Here's how the part is built. I have some questions about the finished solid (model axes, mm). Face numbers are marked on the shaded views. A direction names the side the tool comes from. Round coordinates to 2 decimals unless told otherwise and drop trailing zeros. Loops run counter-clockwise (first coordinate to the right, second up) from the corner with the lowest first, then second, coordinate; pieces in that order, holes last. Notation, with made-up numbers: M -40,-18 L -8,-18 A19 cw -8,-4 Z; hole C -20,77 d3. An arc over 180 degrees is marked long. One line per question, with ' | ' between items. Start each with the question number.
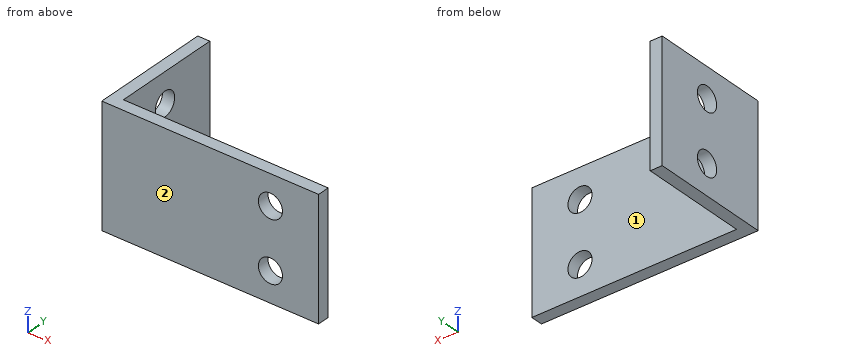
```python
from build123d import *

# Parameters (mm, degrees)
AUFSATZ_LINEAR_AUSTRAGEN1_DEPTH      = 15
AUFSATZ_LINEAR_AUSTRAGEN1_DEPTH_BACK = 15
SKIZZE5_R                            = 3
SCHNITT_LINEAR_AUSTRAGEN1_DEPTH      = 24
SKIZZE7_R                            = 3
SCHNITT_LINEAR_AUSTRAGEN2_DEPTH      = 14


with BuildPart() as part:
    # Skizze2 → Aufsatz-Linear austragen1 (new body, two sides)
    with BuildSketch(Plane.XY) as aufsatz_linear_austragen1_sk:
        Polygon((14, 51), (11, 51), (11, 21), (65, 21), (65, 24), (14, 24), align=None)
    extrude(amount=AUFSATZ_LINEAR_AUSTRAGEN1_DEPTH)
    extrude(aufsatz_linear_austragen1_sk.sketch, amount=-AUFSATZ_LINEAR_AUSTRAGEN1_DEPTH_BACK)

    # Skizze5 → Schnitt-Linear austragen1 (cut)
    with BuildSketch(Plane(origin=(0, 0, 0), x_dir=(1, 0, 0), z_dir=(0, 1, 0))):
        with Locations((53, -7.5)):
            Circle(SKIZZE5_R)
        with Locations((53, 7.5)):
            Circle(SKIZZE5_R)
    extrude(amount=SCHNITT_LINEAR_AUSTRAGEN1_DEPTH, mode=Mode.SUBTRACT)

    # Skizze7 → Schnitt-Linear austragen2 (cut)
    with BuildSketch(Plane(origin=(0, 0, 0), x_dir=(0, 0, -1), z_dir=(1, 0, 0))):
        with Locations((7.5, 37)):
            Circle(SKIZZE7_R)
        with Locations((-7.5, 37)):
            Circle(SKIZZE7_R)
    extrude(amount=SCHNITT_LINEAR_AUSTRAGEN2_DEPTH, mode=Mode.SUBTRACT)


solid = part.part
```
1) Imagine slicing it at B-B (z = -7.5). Write out the boundary of the cut face in (x, y).
2) For the marked faces 1 and 2, which set-ups out of +Z, -Z, +X, -X, +Y, -Y let a thin tool reach every point of the face, with its end or its side?
3) Imagine slicing it at C-C (x = 53). Write out the boundary of the cut face in (y, z), then the cut area to 3 significant figures.
4) Imagine slicing it at D-D (z = 8.75). Write out the boundary of the cut face in (x, y), then the cut area to 3 significant figures.
5) Imagine slicing it at A-A (y = 37). Write out the boundary of the cut face in (x, z).
6) I'm going to push flat-ended pins straight in: pin 1 Ø6 at (x, z) = (43.5, 5) entering from +Y; pin 2 Ø3.5 at (x, z) = (53, 7.5) entering from +Y; pin 3 Ø1 at (y, z) = (25, -11) entering from +X; pin 4 Ø7 at (y, z) = (37, 7.5) entering from -X. Where does each tip first touch, or does it pass through?
7) Please list where these lines run through material, in increasing order: L1, parallel to Z at x = 12.75, y = 37; L2, parallel to X at y = 22.65, z = -7.5; L3, parallel to Y at x = 12.1, z = -7.5. Write a range as from..to.
Results are:
1) outline: M 11,21 L 50,21 L 50,24 L 14,24 L 14,34 L 11,34 Z; M 11,40 L 14,40 L 14,51 L 11,51 Z; M 56,21 L 65,21 L 65,24 L 56,24 Z
2) face 1: +Z, -Z, +X, +Y | face 2: +Z, -Z, +X, -X, -Y
3) outline: M 21,-15 L 24,-15 L 24,-10.5 L 21,-10.5 Z; M 21,-4.5 L 24,-4.5 L 24,4.5 L 21,4.5 Z; M 21,10.5 L 24,10.5 L 24,15 L 21,15 Z | area: 54.0 mm²
4) outline: M 11,21 L 50.27,21 L 50.27,24 L 14,24 L 14,34.27 L 11,34.27 Z; M 11,39.73 L 14,39.73 L 14,51 L 11,51 Z; M 55.73,21 L 65,21 L 65,24 L 55.73,24 Z | area: 210 mm²
5) outline: M 11,-15 L 14,-15 L 14,-10.5 L 11,-10.5 Z; M 11,-4.5 L 14,-4.5 L 14,4.5 L 11,4.5 Z; M 11,10.5 L 14,10.5 L 14,15 L 11,15 Z
6) pin 1: y = 24 | pin 2: through | pin 3: x = 14 | pin 4: x = 11
7) L1: -15..-10.5, -4.5..4.5, 10.5..15 | L2: 11..50, 56..65 | L3: 21..34, 40..51
